Read the model definition and answer for the solid it produces. Units are mm, in the model's axes. A direction names the side the tool comes from. Coordinates: 2 decimals unless noted, no trailing zeros. Write each loop counter-clockwise with the first axis right and the second up, starting at its lowest first coordinate (ties: lowest second). Pieces come first, ordered by that corner, then holes.
Item 1: This flat-tipped pin is pushed along its axis until it touches: P1, Ø1, axis at y = 0.5, z = -16.5, coming from the -X side. Where does it stop, or does it pass through?
Item 2: Section C-C (z = 0) is taken. Give the vertices of the cut face in (x, y).
Item 3: Section A-A (y = 1.6) is taken. Give the vertices of the cut face in (x, z).
Item 4: Straight lines are drawn through the part: probe 1 along X at (y, z) = (1.1, -2); probe 2 along Z at (x, y) = (0, 1.5); probe 3 along X at (y, z) = (1.2, 0). For each, find the intervals that lie inside material, in ascending order.
Item 5: Section D-D (x = -15) is taken. Give the vertices of the cut face in (y, z), then the cut area to 3 significant figures.
Item 6: Determine the mould class of faces 1 (the face through (27.85, 0.99, 1.28)), 2 (the face through (-17.62, 0.99, 30.24)), 3 (the face through (-9.433, 0.986, -24.887)), 4 (the face through (-25, 1, 0)) for opening direction X: released by +X, released by -X, zero draft, split by the parting line, or undercut.
Item 7: A tool of negligible diameter and unlimited length cuts with its end or side. For faces 5 (the face through (-9.45, 0.99, 24.93)), 6 (the face through (12.768, 0.986, -21.494)), 7 (the face through (-15, 1, 23.481)), from which of +Z, -Z, +X, -X, +Y, -Y can it reach the whole face along a straight path? Write none if from no direction.
Item 8: Section B-B (x = 0) is taken. Give the vertices of the cut face in (y, z).
from build123d import *

# Parameters (mm, degrees)
SKETCH1_R           = 25
SKETCH1_W           = 5
SKETCH1_H           = 5
BOSS_EXTRUDE1_DEPTH = 2
CUT_EXTRUDE1_REACH  = 4
SKETCH2_R           = 6.15
FILLET1_R           = 1


with BuildPart() as part:
    # Sketch1 → Boss-Extrude1 (new body)
    with BuildSketch(Plane(origin=(0, 0, 0), x_dir=(1, 0, 0), z_dir=(0, 1, 0))):
        Circle(SKETCH1_R)
        with BuildLine():
            Line((0, 0), (-17.886625066, -21.898189918))
            ThreePointArc((-17.886625066, -21.898189918), (-17.5, -30.310889132), (-10.021076233, -26.439366654))
            Line((-10.021076233, -26.439366654), (0, 0))
        make_face()
        with Locations((-15, -25.980762114)):
            Rectangle(SKETCH1_W, SKETCH1_H, mode=Mode.SUBTRACT)
        with BuildLine():
            Line((0, 0), (27.907701299, -4.541176736))
            ThreePointArc((27.907701299, -4.541176736), (35, 0), (27.907701299, 4.541176736))
            Line((27.907701299, 4.541176736), (0, 0))
        make_face()
        Polygon((29.084936491, -3.415063509), (26.584936491, 0.915063509), (30.915063509, 3.415063509), (33.415063509, -0.915063509), align=None, mode=Mode.SUBTRACT)
        with BuildLine():
            Line((0, 0), (-10.021076233, 26.439366654))
            ThreePointArc((-10.021076233, 26.439366654), (-17.5, 30.310889132), (-17.886625066, 21.898189918))
            Line((-17.886625066, 21.898189918), (0, 0))
        make_face()
        Polygon((-11.584936491, 26.895825623), (-14.084936491, 22.565698604), (-18.415063509, 25.065698604), (-15.915063509, 29.395825623), align=None, mode=Mode.SUBTRACT)
    extrude(amount=BOSS_EXTRUDE1_DEPTH)

    # Sketch2 → Cut-Extrude1 (cut, up to next)
    with BuildSketch(Plane(origin=(0, 0, 0), x_dir=(-1, 0, 0), z_dir=(0, -1, 0)), mode=Mode.PRIVATE) as cut_extrude1_sk1:
        Circle(SKETCH2_R)
    cut_extrude1_tool1 = extrude(cut_extrude1_sk1.sketch, amount=-CUT_EXTRUDE1_REACH, mode=Mode.PRIVATE) & part.part
    add(cut_extrude1_tool1.solids().sort_by_distance((0, 0, 0))[0], mode=Mode.SUBTRACT)

    # Fillet1
    fillet1_edges = [part.edges().sort_by_distance(p)[0] for p in [
        (6.15, 0, 0),
    ]]
    fillet(fillet1_edges, radius=FILLET1_R)


solid = part.part
Established:
1. P1: stops at x = -19.21
2. outline: (-25, 0) - (-7.15, 0) arc R1 ccw to (-6.15, 1) - (-6.15, 2) - (-25, 2) - close; (6.15, 1) arc R1 ccw to (7.15, 0) - (27.11, 0) - (27.11, 2) - (6.15, 2) - close; (32.89, 0) - (35, 0) - (35, 2) - (32.89, 2) - close
3. outline: (-17.89, -21.9) arc R5 ccw (long way) to (-10.02, -26.44) - (-8.86, -23.38) arc R25 ccw to (24.68, -4.02) - (27.91, -4.54) arc R5 ccw (long way) to (27.91, 4.54) - (24.68, 4.02) arc R25 ccw to (-8.86, 23.38) - (-10.02, 26.44) arc R5 ccw (long way) to (-17.89, 21.9) - (-15.82, 19.36) arc R25 ccw to (-15.82, -19.36) - close; hole (-18.42, -25.07) - (-15.92, -29.4) - (-11.58, -26.9) - (-14.08, -22.57) - close; hole (-17.5, 23.48) - (-12.5, 23.48) - (-12.5, 28.48) - (-17.5, 28.48) - close; hole circle Ø12.3 at (0, 0); hole (26.58, -0.92) - (30.92, -3.42) - (33.42, 0.92) - (29.08, 3.42) - close
4. probe 1: x = -24.92 to -5.82, 5.82 to 28.46, 31.73 to 34.58
4. probe 2: z = -25 to -6.15, 6.15 to 25
4. probe 3: x = -25 to -6.15, 6.15 to 27.11, 32.89 to 35
5. outline: (0, -30.98) - (2, -30.98) - (2, -28.87) - (0, -28.87) - close; (0, -23.09) - (2, -23.09) - (2, 23.48) - (0, 23.48) - close; (0, 28.48) - (2, 28.48) - (2, 30.98) - (0, 30.98) - close
5. area: 102 mm2
6. face 1: undercut
6. face 2: split by the parting line
6. face 3: undercut
6. face 4: released by -X
7. face 5: +Z, +Y, -Y
7. face 6: -Z, +Y, -Y
7. face 7: +Y, -Y
8. outline: (0, -25) - (2, -25) - (2, -6.15) - (1, -6.15) arc R1 ccw to (0, -7.15) - close; (0, 7.15) arc R1 ccw to (1, 6.15) - (2, 6.15) - (2, 25) - (0, 25) - close
